Work out the finished part from the listing and answer in its coordinate system (mm). A direction names the side the tool comes from. Coordinates: 2 decimals unless noted, no trailing zeros. Order: outer loops, then holes, each group sorted by start corner. A loop starts at its lowest first (then second) coordinate and runs counter-clockwise, first axis right, second up. Notation, with made-up numbers: M 60,-2.5 L 114,-2.5 A19 ccw 114,17.5 Z; hole C 75,-17.5 d11. An arc over 180 degrees is marked long. Use a Markdown table: item, result. Add a question column.
from build123d import *
from build123d.topology import SkipClean

# Parameters (mm, degrees)
CROQUIS3_R                 = 2.5
SALIENTE_EXTRUIR1_DEPTH    = 5
CROQUIS6_W                 = 27
CROQUIS6_H                 = 16.5
CORTAR_EXTRUIR1_DEPTH      = 2
CROQUIS7_W                 = 29
CROQUIS7_H                 = 18.5
CROQUIS7_W_2               = 27
CROQUIS7_H_2               = 16.5
SALIENTE_EXTRUIR2_DEPTH    = 2.5
CROQUIS8_W                 = 12
CROQUIS8_H                 = 18.5
SALIENTE_EXTRUIR3_DEPTH    = 2
CROQUIS9_W                 = 12.5
CROQUIS9_H                 = 8
CORTAR_EXTRUIR2_DEPTH      = 10
CROQUIS10_R                = 3.25
CORTAR_EXTRUIR3_DEPTH      = 10
CORTAR_EXTRUIR4_DEPTH      = 3
CORTAR_EXTRUIR4_DEPTH_BACK = 3
CROQUIS12_R                = 4.493807468
CROQUIS12_R_2              = 2.5
SALIENTE_EXTRUIR4_DEPTH    = 15
SALIENTE_EXTRUIR5_DEPTH    = 1.4
REDONDEO1_R                = 3
SALIENTE_EXTRUIR6_START    = 10
CROQUIS14_R                = 5.706356105
CROQUIS14_R_2              = 3.25
SALIENTE_EXTRUIR6_DEPTH    = 10
CORTAR_EXTRUIR5_DEPTH      = 10


with BuildPart() as part:
    # Croquis3 → Saliente-Extruir1 (new body)
    with BuildSketch(Plane.XY):
        with BuildLine():
            Line((-8.662935846, -3.067476434), (-11.613388129, -8.280831326))
            ThreePointArc((-11.613388129, -8.280831326), (-19.406371569, -8.331091381), (-15.524316735, -1.57366826))
            Line((-15.524316735, -1.57366826), (-15.524316735, 20.438715392))
            ThreePointArc((-15.524316735, 20.438715392), (-19.406371569, 27.196138513), (-11.613388129, 27.145878458))
            Line((-11.613388129, 27.145878458), (-8.662935846, 21.932523566))
            Line((-8.662935846, 21.932523566), (-8.662935846, -3.067476434))
        make_face()
        with Locations((-15.524316735, 24.93252286)):
            Circle(CROQUIS3_R, mode=Mode.SUBTRACT)
        with Locations((-15.524316735, -6.067475728)):
            Circle(CROQUIS3_R, mode=Mode.SUBTRACT)
    extrude(amount=SALIENTE_EXTRUIR1_DEPTH)

    # Croquis5 → section 0 of recubrir1
    with BuildSketch(Plane(origin=(32.473941286, 0, 18.748838743), x_dir=(0.5000000000000042, 0, -0.8660254037844363), z_dir=(0.8660254037844363, 0, 0.5000000000000042)), mode=Mode.PRIVATE) as recubrir1_s0:
        with BuildLine():
            Line((-4.331467923, 21.932523566), (-9.331467923, 21.932523566))
            Line((-9.331467923, 21.932523566), (-9.331467923, -3.067476434))
            Line((-9.331467923, -3.067476434), (-4.331467923, -3.067476434))
            Line((-4.331467923, -3.067476434), (-4.331467923, 21.932523566))
        make_face()
    # loft up to a face of the part (recubrir1)
    loft([recubrir1_s0.sketch, part.faces().sort_by_distance((-8.662935846, 9.432523566, 2.5))[0]])

    # Croquis6 → Cortar-Extruir1 (cut)
    with BuildSketch(Plane(origin=(-2.165733961, 0, 3.751161257), x_dir=(-0.8660254037844364, 0, -0.5000000000000041), z_dir=(0.500000000000004, 0, -0.8660254037844363))):
        with Locations((-22.997677486, 9.432523566)):
            Rectangle(CROQUIS6_W, CROQUIS6_H)
    extrude(amount=-CORTAR_EXTRUIR1_DEPTH, mode=Mode.SUBTRACT)

    # Croquis7 → Saliente-Extruir2 (add)
    with BuildSketch(Plane(origin=(-2.165733961, 0, 3.751161257), x_dir=(-0.8660254037844364, 0, -0.5000000000000041), z_dir=(0.500000000000004, 0, -0.8660254037844363))):
        with Locations((-22.997677486, 9.432523566)):
            Rectangle(CROQUIS7_W, CROQUIS7_H)
        with Locations((-22.997677486, 9.432523566)):
            Rectangle(CROQUIS7_W_2, CROQUIS7_H_2, mode=Mode.SUBTRACT)
    extrude(amount=SALIENTE_EXTRUIR2_DEPTH)

    # Croquis8 → Saliente-Extruir3 (add)
    with BuildSketch(Plane(origin=(-0.915733961, 0, 1.586097747), x_dir=(-0.8660254037844364, 0, -0.500000000000004), z_dir=(0.500000000000004, 0, -0.8660254037844365))):
        with Locations((-14.497677486, 9.432523566)):
            Rectangle(CROQUIS8_W, CROQUIS8_H)
    extrude(amount=SALIENTE_EXTRUIR3_DEPTH)

    # Croquis9 → Cortar-Extruir2 (cut)
    with BuildSketch(Plane(origin=(0.084266039, 0, -0.14595306), x_dir=(-0.8660254037844364, 0, -0.5000000000000041), z_dir=(0.500000000000004, 0, -0.8660254037844363))):
        with Locations((-9.747677486, 9.182523566)):
            Rectangle(CROQUIS9_W, CROQUIS9_H)
    extrude(amount=-CORTAR_EXTRUIR2_DEPTH, mode=Mode.SUBTRACT)

    # Croquis10 → Cortar-Extruir3 (cut)
    with BuildSketch(Plane(origin=(-2.165733961, 0, 3.751161257), x_dir=(-0.8660254037844364, 0, -0.5000000000000041), z_dir=(0.500000000000004, 0, -0.8660254037844363))):
        with Locations((1.502322514, 15.932523566)):
            Circle(CROQUIS10_R)
        with Locations((1.502322514, 2.932523566)):
            Circle(CROQUIS10_R)
    extrude(amount=-CORTAR_EXTRUIR3_DEPTH, mode=Mode.SUBTRACT)

    # Croquis11 → Cortar-Extruir4 (cut, two sides: drawn at the far end of the back side and taken through both)
    with BuildSketch(Plane(origin=(-4.488412426, 0, 7.498698109), x_dir=(0.8580379698740155, 0, 0.5135862559049632), z_dir=(-0.5135862559049631, 0, 0.8580379698740154)).offset(-CORTAR_EXTRUIR4_DEPTH_BACK)):
        Polygon((-6.099034085, 15.932523566), (-3.731897982, 11.832523566), (1.002374226, 11.832523566), (3.369510329, 15.932523566), (1.002374226, 20.032523566), (-3.731897982, 20.032523566), align=None)
        Polygon((-3.731897982, -1.167476434), (-6.099034085, 2.932523566), (-3.731897982, 7.032523566), (1.002374226, 7.032523566), (3.369510329, 2.932523566), (1.002374226, -1.167476434), align=None)
    extrude(amount=CORTAR_EXTRUIR4_DEPTH + CORTAR_EXTRUIR4_DEPTH_BACK, mode=Mode.SUBTRACT)

    # Croquis12 → Saliente-Extruir4 (add)
    # profile 1 of 2: a face of its own
    with SkipClean():  # the faces are left unmerged after this step: merging them gives an invalid solid
        with BuildSketch(Plane.XY.offset(5)):
            with Locations(Location((-15.524316735, -6.067475728, 0), (0, 0, 90))):
                Circle(CROQUIS12_R)
            with Locations((-15.524316735, -6.067475728)):
                Circle(CROQUIS12_R_2, mode=Mode.SUBTRACT)
        # profile 2 of 2: a face of its own
        with BuildSketch(Plane.XY.offset(5)):
            with Locations(Location((-15.524316735, 24.93252286, 0), (0, 0, 270))):
                Circle(CROQUIS12_R)
            with Locations((-15.524316735, 24.93252286)):
                Circle(CROQUIS12_R_2, mode=Mode.SUBTRACT)
        extrude(amount=SALIENTE_EXTRUIR4_DEPTH)

    # Croquis13 → Saliente-Extruir5 (add)
    with SkipClean():  # the faces are left unmerged after this step: merging them gives an invalid solid
        with BuildSketch(Plane(origin=(0, 21.932523566, 0), x_dir=(1, 0, 0), z_dir=(0, 1, 0))):
            Polygon((-8.662935846, -5), (16.397254921, -20), (-16.030509266, -20), (-16.030509266, -5), align=None)
        saliente_extruir5 = extrude(amount=-SALIENTE_EXTRUIR5_DEPTH)

    # Simetría1: Saliente-Extruir5 across plane
    with SkipClean():  # the faces are left unmerged after this step: merging them gives an invalid solid
        add(saliente_extruir5.mirror(Plane(origin=(0, 9.432523566, 0), x_dir=(0, 0, 1), z_dir=(0, -1, 0))))

    # Redondeo1
    # the kernel refuses this fillet: 3 mm, written as the material it adds along each edge
    with BuildSketch(Plane(origin=(16.397254921, 21.932523566, 20), x_dir=(0.8580379698740132, 0, 0.5135862559049668), z_dir=(0, -1, 0))) as redondeo1_piece_1:
        with BuildLine():
            CenterArc((REDONDEO1_R * 0.2764132188, REDONDEO1_R), REDONDEO1_R, 239.0969949, 30.9030051)
            Line((-REDONDEO1_R * 0.237173037105, REDONDEO1_R * 0.141962030126), (0, 0))
            Line((0, 0), (REDONDEO1_R * 0.2764132188, 0))
        make_face()
    extrude(amount=1.4)
    with BuildSketch(Plane(origin=(-12.178526873, 21.932523566, 20), x_dir=(0.357397896635504, 0.9339522169150398, 0), z_dir=(0, 0, -1))) as redondeo1_piece_2_section:
        with BuildLine():
            CenterArc((4.284349419, 2.80185655), REDONDEO1_R, 159.059522314, 89.999994603)
            Line((1.482492768, 3.87405024), (0, 0))
            ThreePointArc((0, 0), (1.606077732, 0.296806172), (3.212155465, 0))
        make_face()
    redondeo1_piece_2 = extrude(amount=25.370044017, mode=Mode.PRIVATE)
    redondeo1_piece_2 = split(redondeo1_piece_2, bisect_by=Plane(origin=(-10.732886495, 22.627434276, 0), z_dir=(0, 0, 1)), keep=Keep.TOP, mode=Mode.PRIVATE)
    redondeo1_piece_2 = split(redondeo1_piece_2, bisect_by=Plane(origin=(-4.802740059, 22.627434276, 2.228685076), z_dir=(-0.5000000000000042, 0, 0.8660254037844363)), keep=Keep.TOP, mode=Mode.PRIVATE)
    add(redondeo1_piece_2)
    with BuildSketch(Plane(origin=(16.397254921, -3.067476434, 20), x_dir=(0.8580379698740109, 0, 0.5135862559049705), z_dir=(0, 1, 0))) as redondeo1_piece_3:
        with BuildLine():
            CenterArc((REDONDEO1_R * 0.2764132188, -REDONDEO1_R), REDONDEO1_R, 90, 30.9030051)
            Line((-REDONDEO1_R * 0.237173037105, -REDONDEO1_R * 0.141962030126), (0, 0))
            Line((0, 0), (REDONDEO1_R * 0.2764132188, 0))
        make_face()
    extrude(amount=1.4)
    with BuildSketch(Plane(origin=(-12.178526873, -3.067476434, 20), x_dir=(1, 0, 0), z_dir=(0, 0, -1))) as redondeo1_piece_4_section:
        with BuildLine():
            CenterArc((4.148017607, 3), REDONDEO1_R, 180.000005397, 89.999994603)
            ThreePointArc((1.148017607, 2.999999717), (0.851211586, 1.393921957), (0, 0))
            Line((0, 0), (4.148017607, 0))
        make_face()
    redondeo1_piece_4 = extrude(amount=25.370044017, mode=Mode.PRIVATE)
    redondeo1_piece_4 = split(redondeo1_piece_4, bisect_by=Plane(origin=(-8.521402606, -3.090294966, 0), z_dir=(0, 0, 1)), keep=Keep.TOP, mode=Mode.PRIVATE)
    redondeo1_piece_4 = split(redondeo1_piece_4, bisect_by=Plane(origin=(-3.144127143, -3.090294966, 3.18628569), z_dir=(-0.5000000000000042, 0, 0.8660254037844363)), keep=Keep.TOP, mode=Mode.PRIVATE)
    add(redondeo1_piece_4)
    # the kernel refuses this fillet: 3 mm, written as the material it takes off along each edge
    with BuildSketch(Plane(origin=(34.058207325, 21.932523566, 16.004809472), x_dir=(0, -1, 0), z_dir=(-0.5000000000000042, 0, 0.8660254037844363))) as redondeo1_2_piece_1:
        with BuildLine():
            CenterArc((REDONDEO1_R, -REDONDEO1_R), REDONDEO1_R, 90, 90)
            Line((0, -REDONDEO1_R), (0, 0))
            Line((0, 0), (REDONDEO1_R, 0))
        make_face()
    extrude(amount=20, mode=Mode.SUBTRACT)
    with BuildSketch(Plane(origin=(24.058207325, -3.067476434, 33.325317547), x_dir=(-0.8660254037844363, 0, -0.5000000000000041), z_dir=(0.5000000000000042, 0, -0.8660254037844363))) as redondeo1_2_piece_2:
        with BuildLine():
            CenterArc((REDONDEO1_R, REDONDEO1_R), REDONDEO1_R, 180, 90)
            Line((0, REDONDEO1_R), (0, 0))
            Line((0, 0), (REDONDEO1_R, 0))
        make_face()
    extrude(amount=20, mode=Mode.SUBTRACT)

    # Croquis14 → Saliente-Extruir6 (add)
    with BuildSketch(Plane(origin=(-2.165733961, 0, 3.751161257), x_dir=(-0.8660254037844363, 0, -0.5000000000000042), z_dir=(0.5000000000000041, 0, -0.8660254037844362)).offset(SALIENTE_EXTRUIR6_START)):
        with Locations(Location((1.502322514, 15.932523566, 0), (0, 0, 208.810793743))):
            Circle(CROQUIS14_R)
        with Locations((1.502322514, 15.932523566)):
            Circle(CROQUIS14_R_2, mode=Mode.SUBTRACT)
    extrude(amount=-SALIENTE_EXTRUIR6_DEPTH)

    # Croquis15 → Cortar-Extruir5 (cut)
    with BuildSketch(Plane(origin=(-2.947653659, 0, 4.9245842), x_dir=(0.8580379698740153, 0, 0.5135862559049633), z_dir=(-0.5135862559049633, 0, 0.8580379698740153))):
        Polygon((3.369510329, 15.932523566), (1.002374226, 20.032523566), (-3.731897982, 20.032523566), (-6.099034085, 15.932523566), (-3.731897982, 11.832523566), (1.002374226, 11.832523566), align=None)
    extrude(amount=-CORTAR_EXTRUIR5_DEPTH, mode=Mode.SUBTRACT)


solid = part.part
(1) A cutting plane is placed at D-D on y = 24. Write down the section's boundary in (x, z).
(2) A cutting plane is placed at A-A on y = 8. Write down the section's boundary in (x, z).
(3) Given P1, Ø4, axis at x = -13, z = 1, coming from the -Y side; P2, Ø0.9, axis at x = -10, y = 24.5, coming from the +Z side; P3, Ø12, axis at x = -3, z = 1, coming from the -Y side, each flat-ended and moving along its own axis, determine where each tip first touches the part or whether it passes through.
(4) A cutting plane is placed at B-B on z = 11. Write down the section's boundary in (x, y), plus the area to 3 significant figures.
(5) Which of the six approach directions +Z, -Z, +X, -X, +Y, -Y give full straight-line access (tool end or side, diameter ignored) to faces 4 (the flat face through (-9, -3, 20)), 5 (the flat face through (-10.2, 23.8, 5)), 6 (the flat face through (0.665, 13.854, 3.114))?
(6) A cutting plane is placed at C-C on x = -9.5. Write down the section's boundary in (y, z).
(7) The mould has two halves that part along Y. Classify faces 1 (the flat face through (-4, 20.533, 15)), 2 (the flat face through (15.022, 9.562, 8.478)), 3 (the flat face through (4, -3.067, 12)): pulls with the +Y half, pulls with the -Y half, needs draft (parallel to the pull), parting line crosses it, or undercut.
(8) Straight lines are drawn through the part: line 1 (Y direction, x = 5, z = 14); line 2 (Y direction, x = 1, z = 9); line 3 (X direction, y = 17.5, z = 2). For each, find the intervals that lie inside material, in ascending order.
From the geometry:
| question | item | result |
|---|---|---|
| 1 | outline | M -19.92,0 L -17.84,0 L -17.84,20 L -19.92,20 Z; M -13.2,0 L -9.83,0 L -9.83,5 L -10.88,5 L -10.88,20 L -13.2,20 Z |
| 2 | outline | M -15.52,0 L -8.66,0 L 0.86,5.5 L -1.37,9.37 L -8.66,5 L -15.52,5 Z; M 9.36,15.79 L 10.69,13.48 L 28.44,23.73 L 30.69,19.83 L 31.56,20.33 L 27.81,26.83 Z; M 12.94,9.58 L 13.94,7.85 L 17.84,10.1 L 16.84,11.83 Z |
| 3 | P1 | stops at y = -10.53 |
| 3 | P2 | stops at z = 5 |
| 3 | P3 | stops at y = -3.66 |
| 4 | outline | M -14.61,-1.67 A4.49 ccw long -11.03,-6.07 A3 cw -8.03,-3.07 L 10.39,-3.07 L 10.39,0.18 L 17.32,0.18 L 17.32,18.68 L 10.39,18.68 L 10.39,21.93 L -8.03,21.93 A3 cw -11.03,24.93 A4.49 ccw long -14.61,20.53 L 1.36,20.53 L 1.36,13.18 L 6.39,13.18 L 6.39,17.68 L 15.39,17.68 L 15.39,1.18 L 6.39,1.18 L 6.39,5.18 L 1.36,5.18 L 1.36,-1.67 Z; hole C -15.52,-6.07 d5; hole C -15.52,24.93 d5 |
| 4 | area | 299 mm2 |
| 5 | face 4 | +Z, -X, +Y, -Y |
| 5 | face 5 | +Z, +X, +Y |
| 5 | face 6 | none |
| 6 | outline | M -4.55,0 L 23.41,0 L 23.41,5 L 22.32,5 L 22.32,20 L 20.53,20 L 20.53,5 L 16.83,5 L 15.93,4 L 15.04,5 L 3.83,5 L 2.93,4 L 2.04,5 L -1.67,5 L -1.67,20 L -3.45,20 L -3.45,5 L -4.55,5 Z |
| 7 | face 1 | undercut |
| 7 | face 2 | needs draft |
| 7 | face 3 | pulls with the -Y half |
| 8 | line 1 | y = -3.07 to -1.67, 20.53 to 21.93 |
| 8 | line 2 | y = -3.07 to 5.18, 13.18 to 21.93 |
| 8 | line 3 | x = -15.52 to -7.25, 1.68 to 3.45 |
